Here's how the part is built. I have some questions about the finished solid (model axes, mm). Face numbers are marked on the shaded views. A direction names the side the tool comes from. Round coordinates to 2 decimals unless told otherwise and drop trailing zeros. Order: outer loops, then holes, each group sorted by start corner. A loop starts at its lowest first (then second) coordinate and runs counter-clockwise, first axis right, second up.
```python
from build123d import *

# Parameters (mm, degrees)
BOSS_EXTRUDE1_DEPTH     = 2
SKETCH2_W               = 3.5
SKETCH2_H               = 2
CUT_EXTRUDE1_DEPTH      = 22
BOSS_EXTRUDE2_DEPTH     = 7
BOSS_EXTRUDE3_DEPTH     = 6
SKETCH5_R               = 2.25
CUT_EXTRUDE3_DEPTH      = 37
CUT_EXTRUDE3_DEPTH_BACK = 37
FILLET1_R               = 3
FILLET2_R               = 0.5
CUT_EXTRUDE4_DEPTH      = 37
FILLET3_R               = 0.5
FILLET4_R               = 0.5
CUT_EXTRUDE5_DEPTH      = 10
FILLET8_R               = 1
SKETCH8_W               = 0.1
SKETCH8_H               = 1
CUT_EXTRUDE6_DEPTH      = 0.1
SKETCH10_R              = 57.556720945
CUT_EXTRUDE7_DEPTH      = 11
CUT_EXTRUDE7_DEPTH_BACK = 1


with BuildPart() as part:
    # Sketch1 → Boss-Extrude1 (new body)
    with BuildSketch(Plane(origin=(0, 0, 0), x_dir=(1, 0, 0), z_dir=(0, 1, 0))):
        with BuildLine():
            Line((-27.424590139, -24.837307739), (27.424590139, -24.837307739))
            ThreePointArc((27.424590139, -24.837307739), (37, 0), (27.424590139, 24.837307739))
            Line((27.424590139, 24.837307739), (-27.424590139, 24.837307739))
            ThreePointArc((-27.424590139, 24.837307739), (-37, 0), (-27.424590139, -24.837307739))
        make_face()
    extrude(amount=BOSS_EXTRUDE1_DEPTH)

    # Sketch2 → Cut-Extrude1 (cut)
    with BuildSketch(Plane.XZ):
        Polygon((-8, 0), (-8, 9.5), (-11, 9.5), (-11, -9.5), (-8, -9.5), align=None)
        with Locations((-9.75, 0)):
            Rectangle(SKETCH2_W, SKETCH2_H)
    extrude(amount=-CUT_EXTRUDE1_DEPTH, mode=Mode.SUBTRACT)

    # Sketch3 → Boss-Extrude2 (add)
    with BuildSketch(Plane(origin=(0, 2, 0), x_dir=(1, 0, 0), z_dir=(0, 1, 0))):
        Polygon((2.9, 11.6), (2.9, 10.1), (19, 10.1), (20.5, 10.1), (20.5, 11.6), align=None)
        Polygon((20.5, 10.1), (19, 10.1), (19, -10.1), (19, -11.6), (20.5, -11.6), align=None)
        Polygon((19, -11.6), (19, -10.1), (-14.6, -10.1), (-16.1, -10.1), (-16.1, -11.6), align=None)
        Polygon((-14.6, 10.1), (2.9, 10.1), (2.9, 11.6), (-16.1, 11.6), (-16.1, 10.1), align=None)
    extrude(amount=BOSS_EXTRUDE2_DEPTH)

    # Sketch4 → Boss-Extrude3 (add)
    with BuildSketch(Plane.XZ):
        Polygon((-8, 0), (-8.02303658, 9.318964787), (-3, 9.318964787), (-3, -9.5), (-8, -9.5), align=None)
    extrude(amount=BOSS_EXTRUDE3_DEPTH)

    # Sketch5 → Cut-Extrude3 (cut, two sides)
    with BuildSketch(Plane.ZY.offset(8)) as cut_extrude3_sk:
        with Locations((-5.031035213, -2.35)):
            Circle(SKETCH5_R)
        with Locations((5.031035213, -2.35)):
            Circle(SKETCH5_R)
    extrude(amount=CUT_EXTRUDE3_DEPTH, mode=Mode.SUBTRACT)
    extrude(cut_extrude3_sk.sketch, amount=-CUT_EXTRUDE3_DEPTH_BACK, mode=Mode.SUBTRACT)

    # Fillet1
    fillet1_edges = [part.edges().sort_by_distance(p)[0] for p in [
        (-5.5, -6, -9.5),
        (-5.51151829, -6, 9.318964787),
    ]]
    fillet(fillet1_edges, radius=FILLET1_R)

    # Fillet2
    fillet2_edges = [part.edges().sort_by_distance(p)[0] for p in [
        (-37, 2, 0),
        (37, 2, 0),
    ]]
    fillet(fillet2_edges, radius=FILLET2_R)

    # Sketch6 → Cut-Extrude4 (cut)
    with BuildSketch(Plane.XZ):
        with BuildLine():
            Line((-34.696885188, 1.668964787), (-31.296885188, 1.668964787))
            ThreePointArc((-31.296885188, 1.668964787), (-29.596885188, -0.031035213), (-31.296885188, -1.731035213))
            Line((-31.296885188, -1.731035213), (-34.696885188, -1.731035213))
            ThreePointArc((-34.696885188, -1.731035213), (-36.396885188, -0.031035213), (-34.696885188, 1.668964787))
        make_face()
        with BuildLine():
            Line((31.302827177, 1.806746588), (34.702827177, 1.806746588))
            ThreePointArc((34.702827177, 1.806746588), (36.402827177, 0.106746588), (34.702827177, -1.593253412))
            Line((34.702827177, -1.593253412), (31.302827177, -1.593253412))
            ThreePointArc((31.302827177, -1.593253412), (29.602827177, 0.106746588), (31.302827177, 1.806746588))
        make_face()
    extrude(amount=-CUT_EXTRUDE4_DEPTH, mode=Mode.SUBTRACT)

    # Fillet3
    fillet3_edges = [part.edges().sort_by_distance(p)[0] for p in [
        (20.5, 9, 0),
        (2.2, 9, -11.6),
        (2.2, 9, 11.6),
        (1.45, 9, -10.1),
        (19, 9, 0),
        (1.45, 9, 10.1),
    ]]
    fillet(fillet3_edges, radius=FILLET3_R)

    # Fillet4
    fillet4_edges = [part.edges().sort_by_distance(p)[0] for p in [
        (-16.1, 9, -10.85),
        (-16.1, 9, 10.85),
        (-16.1, 5.25, -10.1),
        (-16.1, 5.25, -11.6),
        (-16.1, 8.853553391, -11.453553391),
        (-16.1, 8.853553391, -10.246446609),
        (-16.1, 5.25, 11.6),
        (-16.1, 5.25, 10.1),
        (-16.1, 8.853553391, 10.246446609),
        (-16.1, 8.853553391, 11.453553391),
    ]]
    fillet(fillet4_edges, radius=FILLET4_R)

    # Sketch7 → Cut-Extrude5 (cut)
    with BuildSketch(Plane.XZ):
        Polygon((-19.996885188, 19.968964787), (-10.996885188, 19.968964787), (-10.996885188, 11.968964787), (-28.996885188, 11.968964787), (-28.996885188, 19.968964787), align=None)
        Polygon((11.003114812, 11.968964787), (20.003114812, 11.968964787), (20.003114812, 14.968964787), (20.003114812, 19.968964787), (11.003114812, 19.968964787), align=None)
        Polygon((20.003114812, 14.968964787), (20.003114812, 11.968964787), (29.003114812, 11.968964787), (29.003114812, 19.968964787), (20.003114812, 19.968964787), align=None)
        Polygon((-28.996885188, -12.031035213), (-28.996885188, -20.031035213), (-19.996885188, -20.031035213), (-10.996885188, -20.031035213), (-10.996885188, -12.031035213), align=None)
        Polygon((20.003114812, -20.031035213), (11.003114812, -20.031035213), (11.003114812, -12.031035213), (29.003114812, -12.031035213), (29.003114812, -20.031035213), align=None)
    extrude(amount=-CUT_EXTRUDE5_DEPTH, mode=Mode.SUBTRACT)

    # Fillet8
    fillet8_edges = [part.edges().sort_by_distance(p)[0] for p in [
        (11.003114812, 0, 15.968964787),
        (20.003114812, 0, 11.968964787),
        (29.003114812, 0, 15.968964787),
        (20.003114812, 0, 19.968964787),
        (-28.996885188, 0, -16.031035213),
        (-19.996885188, 0, -20.031035213),
        (-10.996885188, 0, -16.031035213),
        (-19.996885188, 0, -12.031035213),
        (20.003114812, 0, -20.031035213),
        (11.003114812, 0, -16.031035213),
        (20.003114812, 0, -12.031035213),
        (29.003114812, 0, -16.031035213),
        (-19.996885188, 0, 19.968964787),
        (-10.996885188, 0, 15.968964787),
        (-19.996885188, 0, 11.968964787),
        (-28.996885188, 0, 15.968964787),
    ]]
    fillet(fillet8_edges, radius=FILLET8_R)

    # Sketch8 → Cut-Extrude6 (cut)
    with BuildSketch(Plane.XY.offset(24.837307739)):
        with Locations((-0.05, 0.5)):
            Rectangle(SKETCH8_W, SKETCH8_H)
        with Locations((0.05, 0.5)):
            Rectangle(SKETCH8_W, SKETCH8_H)
    extrude(amount=-CUT_EXTRUDE6_DEPTH, mode=Mode.SUBTRACT)

    # Sketch10 → Cut-Extrude7 (cut, two sides)
    with BuildSketch(Plane.XZ) as cut_extrude7_sk:
        Circle(SKETCH10_R)
    extrude(amount=CUT_EXTRUDE7_DEPTH, mode=Mode.SUBTRACT)
    extrude(cut_extrude7_sk.sketch, amount=-CUT_EXTRUDE7_DEPTH_BACK, mode=Mode.SUBTRACT)


solid = part.part
```
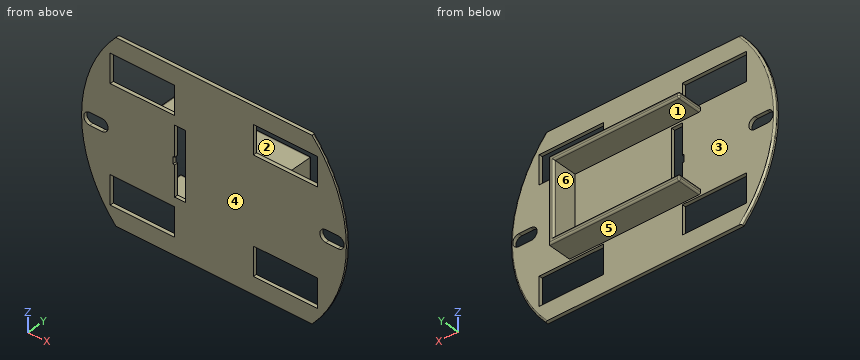
1) If we section it at C-C (x = -4): Write out the boundary of the cut face in (y, z), plus the area to 3 significant figures.
2) For the marked faces 1, 2 and 3, which set-ups out of +Z, -Z, +X, -X, +Y, -Y let a thin tool reach every point of the face, with its end or its side?
3) We'd pull the mould along Z, two halves only. Please class the marked faces 4, 5 and 6: +Z half, -Z half, draft (parallel to the pull), parting line (faces both ways), or undercut.
4) I'm going to push flat-ended pins straight in: pin 1 (1.1 mm diameter, centred on y = 1.5, z = -7, fed in from +X); pin 2 (0.5 mm diameter, centred on x = 33.5, y = 1.5, fed in from +Z); pin 3 (3 mm diameter, centred on x = -0.5, z = 6.5, fed in from +Y); pin 4 (3 mm diameter, centred on x = 22.5, y = 5.5, fed in from -Z). Where does each tip first touch, or does it pass through?
5) If we section it at A-A (x = 23.5): Write out the boundary of the cut face in (y, z).
6) I need wall thicknesses on line 1 (Z direction, x = -7.5, y = 3.75); line 2 (Y direction, x = 34.5, z = -9); line 3 (X direction, y = 8, z = 4). Which ranges of each line are inside material? Lowest first, please.
7) If we section it at B-B (y = 3): Write out the boundary of the cut face in (x, z), plus the area to 3 significant figures.
8) If we section it at D-D (z = 13): Give the number of separate pieces and of enclosed holes in the cut face, plus the area to 3 significant figures.
Solutions:
1. outline: (1, -24.84) - (2, -24.84) - (2, -11.6) - (8.5, -11.6) arc R0.5 ccw to (9, -11.1) - (9, -10.6) arc R0.5 ccw to (8.5, -10.1) - (2, -10.1) - (2, 10.1) - (8.5, 10.1) arc R0.5 ccw to (9, 10.6) - (9, 11.1) arc R0.5 ccw to (8.5, 11.6) - (2, 11.6) - (2, 24.84) - (1, 24.84) - close
1. area: 70.5 mm2
2. face 1: -X, +Y
2. face 2: +Z, +X, -X, +Y
2. face 3: +Y
3. face 4: draft
3. face 5: -Z half
3. face 6: undercut
4. pin 1: stops at x = 36.43
4. pin 2: stops at z = 16.23
4. pin 3: stops at y = 2
4. pin 4: passes through
5. outline: (1, -24.84) - (2, -24.84) - (2, -20.03) - (1, -20.03) - close; (1, -12.03) - (2, -12.03) - (2, 11.97) - (1, 11.97) - close; (1, 19.97) - (2, 19.97) - (2, 24.84) - (1, 24.84) - close
6. line 1: z = -11.6 to -10.1, 10.1 to 11.6
6. line 2: y = 1 to 2
6. line 3: x = 19 to 20.5
7. outline: (-16.1, -11.1) arc R0.5 ccw to (-15.6, -11.6) - (20.5, -11.6) - (20.5, 11.6) - (-15.6, 11.6) arc R0.5 ccw to (-16.1, 11.1) - (-16.1, 10.6) arc R0.5 ccw to (-15.6, 10.1) - (19, 10.1) - (19, -10.1) - (-15.6, -10.1) arc R0.5 ccw to (-16.1, -10.6) - close
7. area: 140 mm2
8. separate pieces: 3
8. enclosed holes: 0
8. area: 33.2 mm2
